The drawing under review shows one solid part. Ordinate dimensions are in mm from its lowest x, y, z. A direction names the side the tool comes from. Give positions to 0.01 mm unless a question says otherwise; leave off trailing zeros. Loops run counter-clockwise (first coordinate to the right, second up) from the corner with the lowest first, then second, coordinate; pieces in that order, holes last. Notation, with made-up numbers: (42, 46.5) -> (76, 46.5) arc R12 ccw to (76, 62.5) -> close; hole circle Ø8 at (-4.75, -4.75). An arc over 180 degrees is marked (long way). Answer in a Markdown table with one row per item. Add a question column.
(1) For the marked faces 1 and 2, list the 3-axis set-ups (+Z, -Z, +X, -X, +Y, -Y) from which the entire face can be reached by the end or side of a thin tool; tool diameter is ignored.
(2) Draft analysis for pull direction Y (two halves, no side actions). For the marked faces 3, 4, 5 and 6, state which applies: +Y half, -Y half, draft (parallel to the pull), parting line (faces both ways), or undercut.
(3) For line 1 (Y direction, x = 4, z = 1.85); line 2 (X direction, y = 24.75, z = 2.5); line 3 (X direction, y = 14.5, z = 5), list the stretches that pass through material, from the lowest coordinate up.
(4) Consider section A-A on x = 9. Write out the cut boundary in (y, z).
(5) Consider section C-C on z = 1.75. Write out the cut boundary in (x, y).
(6) Consider section D-D on y = 4. Write out the cut boundary in (x, z), then the cut area to 3 significant figures.
(7) Consider section B-B on y = 14. Write out the cut boundary in (x, z), then the cut area to 3 significant figures.
(8) For pin 1 (1 mm diameter, centred on x = 6.5, z = 3, fed in from -Y); pin 2 (2 mm diameter, centred on x = 14, y = 24, fed in from +Z); pin 3 (1 mm diameter, centred on x = 10, z = 1.5, fed in from -Y); pin 4 (4 mm diameter, centred on y = 18, z = 7, fed in from -X), all flat-tipped, find the tip position at first contact; note any pin that passes through.
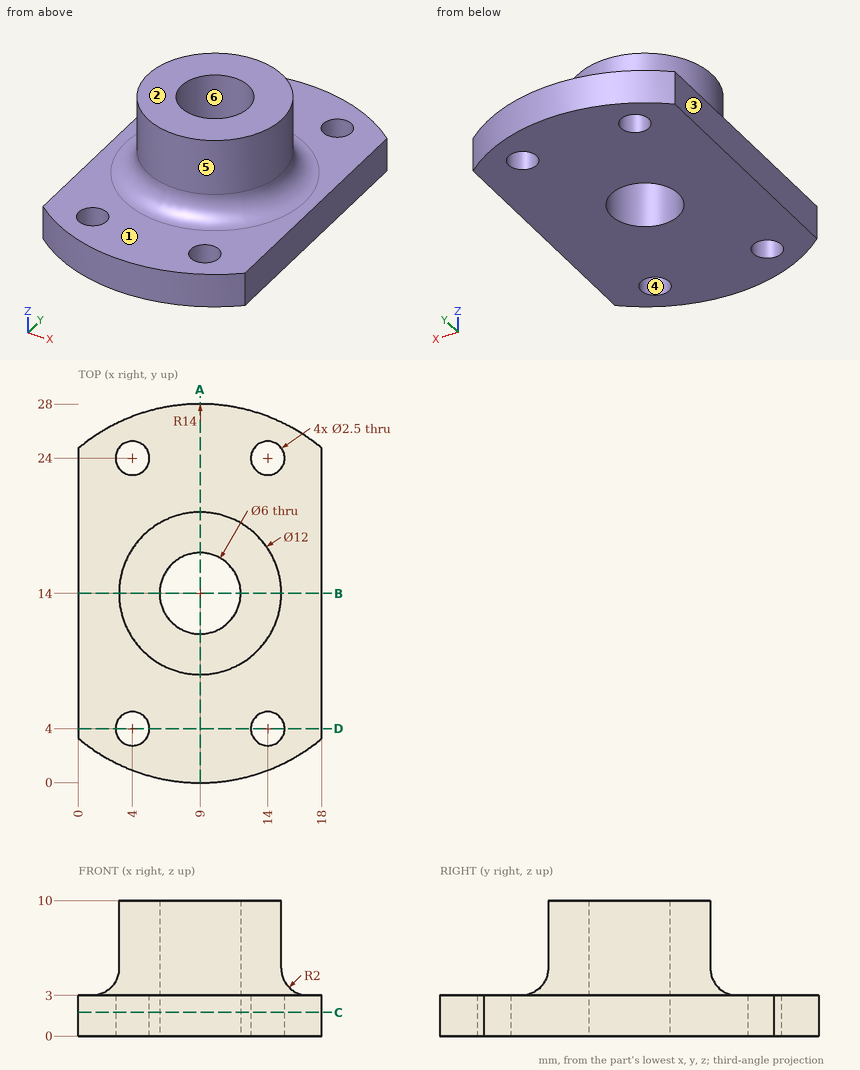
Values follow:
| question | item | result |
|---|---|---|
| 1 | face 1 | +Z |
| 1 | face 2 | +Z, +X, -X, +Y, -Y |
| 2 | face 3 | draft |
| 2 | face 4 | undercut |
| 2 | face 5 | parting line |
| 2 | face 6 | undercut |
| 3 | line 1 | 0.92 to 2.75, 5.25 to 22.75, 25.25 to 27.08 |
| 3 | line 2 | 0.03 to 3, 5 to 13, 15 to 17.97 |
| 3 | line 3 | 3.02 to 6.04, 11.96 to 14.98 |
| 4 | outline | (0, 0) -> (11, 0) -> (11, 10) -> (8, 10) -> (8, 5) arc R2 cw to (6, 3) -> (0, 3) -> close; (17, 0) -> (28, 0) -> (28, 3) -> (22, 3) arc R2 cw to (20, 5) -> (20, 10) -> (17, 10) -> close |
| 5 | outline | (0, 3.28) arc R14 ccw to (18, 3.28) -> (18, 24.72) arc R14 ccw to (0, 24.72) -> close; hole circle Ø2.5 at (4, 4); hole circle Ø2.5 at (4, 24); hole circle Ø6 at (9, 14); hole circle Ø2.5 at (14, 4); hole circle Ø2.5 at (14, 24) |
| 6 | outline | (0, 0) -> (2.75, 0) -> (2.75, 3) -> (0, 3) -> close; (5.25, 0) -> (12.75, 0) -> (12.75, 3) -> (5.25, 3) -> close; (15.25, 0) -> (18, 0) -> (18, 3) -> (15.25, 3) -> close |
| 6 | area | 39.0 mm2 |
| 7 | outline | (0, 0) -> (6, 0) -> (6, 10) -> (3, 10) -> (3, 5) arc R2 cw to (1, 3) -> (0, 3) -> close; (12, 0) -> (18, 0) -> (18, 3) -> (17, 3) arc R2 cw to (15, 5) -> (15, 10) -> (12, 10) -> close |
| 7 | area | 79.7 mm2 |
| 8 | pin 1 | y = 0.14 |
| 8 | pin 2 | through |
| 8 | pin 3 | y = 0.01 |
| 8 | pin 4 | x = 3.34 |
